from build123d import *

# Parameters (mm, degrees)
F1_DEPTH    = 5.08
F3_D        = 3.937
F3_DEPTH    = 12.7
F3_TIP      = 1.1827941286
F4_D        = 3.937
F4_DEPTH    = 12.7
F4_START    = 1.016
F4_TIP      = 1.1827941286
F5_T1_DEPTH = 28.5747319519
F6_SIZE     = 1


# Not quite as in the source:
# - a fillet or chamfer that OpenCascade refuses, or shapes differently, is made with other operations: its cross-section is extruded or revolved along the edge and cut away or added


with BuildPart() as f1:
    # F0 (on Top) → F1 (new body, symmetric)
    with BuildSketch(Plane.XY):
        Polygon((-12.7, -10.16), (12.7, -10.16), (22.225, -9.144), (22.225, 9.144), (12.7, 10.16), (-12.7, 10.16), (-22.225, 9.144), (-22.225, -9.144), align=None)
        with BuildLine():
            ThreePointArc((6.0107370596, -1.016), (0, -6.096), (-6.0107370596, -1.016))
            Line((-6.0107370596, -1.016), (-12.7, -1.016))
            Line((-12.7, -1.016), (-20.32, 0))
            Line((-20.32, 0), (-12.7, 1.016))
            Line((-12.7, 1.016), (-6.0107370596, 1.016))
            ThreePointArc((-6.0107370596, 1.016), (0, 6.096), (6.0107370596, 1.016))
            Line((6.0107370596, 1.016), (12.7, 1.016))
            Line((12.7, 1.016), (20.32, 0))
            Line((20.32, 0), (12.7, -1.016))
            Line((12.7, -1.016), (6.0107370596, -1.016))
        make_face(mode=Mode.SUBTRACT)
    extrude(amount=F1_DEPTH, both=True)

    # F3 (one way)
    with BuildSketch(Plane.XZ):
        with Locations((-11.43, 0), (11.43, 0)):
            Circle(F3_D / 2)
    extrude(amount=-F3_DEPTH, mode=Mode.SUBTRACT)
    with Locations(Plane.XZ):
        with Locations((-11.43, 0), (11.43, 0)):
            with Locations((0, 0, -(F3_DEPTH + F3_TIP / 2))):  # 118° drill point
                Cone(0, F3_D / 2, F3_TIP, mode=Mode.SUBTRACT)

    # F4
    # its depths count from where the whole tool has entered the part; down to there all is cleared
    with Locations(Plane(origin=(0, 0, 0), x_dir=(1, 0, 0), z_dir=(0, 1, 0)).offset(-F4_START)):
        with Locations((-11.43, 0), (11.43, 0)):
            Hole(F4_D / 2, depth=F4_DEPTH)
            with Locations((0, 0, -(F4_DEPTH + F4_TIP / 2))):  # 118° drill point
                Cone(0, F4_D / 2, F4_TIP, mode=Mode.SUBTRACT)

    # F5: chamfer of 2 on 4 edges, made by hand

    # F5_s2 → F5_t1 (cut)
    with BuildSketch(Plane.XZ.offset(-14.2873659759)):
        Polygon((20.225, -5.08), (22.225, -3.08), (22.225, -5.08), align=None)
        Polygon((22.225, 3.08), (20.225, 5.08), (22.225, 5.08), align=None)
        Polygon((-22.225, 3.08), (-20.225, 5.08), (-22.225, 5.08), align=None)
        Polygon((-20.225, -5.08), (-22.225, -3.08), (-22.225, -5.08), align=None)
    extrude(amount=F5_T1_DEPTH, mode=Mode.SUBTRACT)

    # F6
    f6_edges = [f1.edges().sort_by_distance(p)[0] for p in [
        (0, -6.096, -5.08),
        (0, -6.096, 5.08),
        (0, 6.096, 5.08),
        (0, 6.096, -5.08),
    ]]
    chamfer(f6_edges, length=F6_SIZE)


solid = f1.part
Read the model definition and answer for the solid it produces. Units are mm, in the model's axes. A direction names the side the tool comes from. Give positions to 0.01 mm unless a question says otherwise; leave off trailing zeros. Write each loop counter-clockwise with the first axis right and the second up, starting at its lowest first coordinate (ties: lowest second). Pieces come first, ordered by that corner, then holes. Notation, with made-up numbers: (52, -24.75) -> (92, -24.75) arc R22 ccw to (92, -3.75) -> close; hole circle Ø9 at (64.25, 88). An arc over 180 degrees is marked (long way). Answer as a JSON object with one key per item and string values. Group by question number.
1) Find section D-D (x = -16). Write down the section's boundary in (y, z).
2) Find section C-C (z = 0). Write down the section's boundary in (x, y) (1 decimal).
3) A tool of negligible diameter and unlimited length cuts with its end or side. For faces 4 (the conical face through (0.125, -6.254, -4.24)), 5 (the flat face through (-9, -1.016, 0)), 6 (the conical face through (-0.125, 6.254, 4.24)), from which of +Z, -Z, +X, -X, +Y, -Y can it reach the whole face along a straight path? Write none if from no direction.
4) Consider L1, parallel to X at y = -8.25, z = -1.5 (3 decimals); L2, parallel to Y at x = -8.5, z = -2.25; L3, parallel to Z at x = 11.43, y = 4.25. Determine where each line is inside the solid, lowest interval first. Write a range as from..to.
5) Find section A-A (x = 11.43). Write down the section's boundary in (y, z), and give its area (3 significant figures).
6) The mould has two halves that part along Z. Classify faces 1 (the flat face through (-21.239, 0.131, 4.066)), 2 (the flat face through (-0.3, 7.4, -5.08)), 3 (the cylindrical face through (-13.31, -5.61, -0.59)): +Z half, -Z half, draft (parallel to the pull), parting line (faces both ways), or undercut.
7) Find section B-B (z = 2.5). Write down the section's boundary in (x, y) (3 decimals), and give its area (3 significant figures).
8) Each of these flat-tipped pins is pushed along its axis until it touches: P1, Ø3, axis at x = -1.5, y = 4.5, coming from the +Z side; P2, Ø4.5, axis at x = -11.43, z = 0, coming from the +Y side. Where does it stop, or does it pass through?
Values follow:
{
 "1": {"outline": "(-9.81, -5.08) -> (-0.58, -5.08) -> (-0.58, 5.08) -> (-9.81, 5.08) -> close; (0.58, -5.08) -> (9.81, -5.08) -> (9.81, 5.08) -> (0.58, 5.08) -> close"},
 "2": {"outline": "(-22.2, -9.1) -> (-13.4, -10.1) -> (-13.4, -0.9) -> (-20.3, 0) -> (-13.4, 0.9) -> (-13.4, 10.1) -> (-22.2, 9.1) -> close; (-9.5, -10.2) -> (9.5, -10.2) -> (9.5, -1) -> (6, -1) arc R6.1 cw to (-6, -1) -> (-9.5, -1) -> close; (-9.5, 1) -> (-6, 1) arc R6.1 cw to (6, 1) -> (9.5, 1) -> (9.5, 10.2) -> (-9.5, 10.2) -> close; (13.4, -10.1) -> (22.2, -9.1) -> (22.2, 9.1) -> (13.4, 10.1) -> (13.4, 0.9) -> (20.3, 0) -> (13.4, -0.9) -> close"},
 "3": {"face 4": "-Z", "face 5": "+Z, -Z", "face 6": "+Z"},
 "4": {"L1": "x = -22.225..-12.705, -10.155..10.155, 12.705..22.225", "L2": "y = -10.16..-1.02, 1.02..10.16", "L3": "z = -5.08..-1.97, 1.97..5.08"},
 "5": {"outline": "(-10.16, -5.08) -> (-1.02, -5.08) -> (-1.02, -1.97) -> (-10.16, -1.97) -> close; (-10.16, 1.97) -> (-1.02, 1.97) -> (-1.02, 5.08) -> (-10.16, 5.08) -> close; (1.02, -5.08) -> (10.16, -5.08) -> (10.16, -1.97) -> (1.02, -1.97) -> close; (1.02, 1.97) -> (10.16, 1.97) -> (10.16, 5.08) -> (1.02, 5.08) -> close", "area": "114 mm2"},
 "6": {"face 1": "+Z half", "face 2": "-Z half", "face 3": "undercut"},
 "7": {"outline": "(-22.225, -9.144) -> (-12.7, -10.16) -> (12.7, -10.16) -> (22.225, -9.144) -> (22.225, 9.144) -> (12.7, 10.16) -> (-12.7, 10.16) -> (-22.225, 9.144) -> close; hole (-20.32, 0) -> (-12.7, -1.016) -> (-6.011, -1.016) arc R6.096 ccw to (6.011, -1.016) -> (12.7, -1.016) -> (20.32, 0) -> (12.7, 1.016) -> (6.011, 1.016) arc R6.096 ccw to (-6.011, 1.016) -> (-12.7, 1.016) -> close", "area": "725 mm2"},
 "8": {"P1": "stops at z = 4.23", "P2": "stops at y = 10.16"}
}
